Study the drawing (mm; zero at the part's minimum x, y, z) and answer. Give positions to 0.01 mm unless a question says otherwise; leave off trailing zeros. Loops run counter-clockwise (first coordinate to the right, second up) from the corner with the lowest first, then second, coordinate; pieces in that order, holes last. Notation, with made-up numbers: (-11.75, 30) - (22.25, 30) arc R12 cw to (22.25, 43) - close; hole circle Ø6 at (-39.5, -18.5). An arc over 180 degrees is marked (long way). Write item = value, one per line. Start each with the question number.
1) The part is cut by section B-B on x = 25.4. Write down the section's boundary in (y, z).
2) Flat-ended cylindrical pins translate along their axes: P1, Ø1, axis at x = 39, y = 3.5, coming from the -Z side; P2, Ø6, axis at x = 13.5, y = 12.5, coming from the +Z side; P3, Ø1.5, axis at y = 11.5, z = 26.5, coming from the -X side (1 decimal). Find the tip coordinate at first contact, or state that the pin passes through.
3) The mould has two halves that part along Y. Classify the marked faces 1, 2 and 3: +Y half, -Y half, draft (parallel to the pull), parting line (faces both ways), or undercut.
4) The part is cut by section A-A on z = 25.4. Write down the section's boundary in (x, y).
5) Consider probe 1 along Z at (x, y) = (28.5, 14.25); probe 2 along Z at (x, y) = (7.5, 8) (1 decimal); probe 3 along X at (y, z) = (8.75, 14.5) (1 decimal). Determine where each line is inside the solid, lowest interval first.
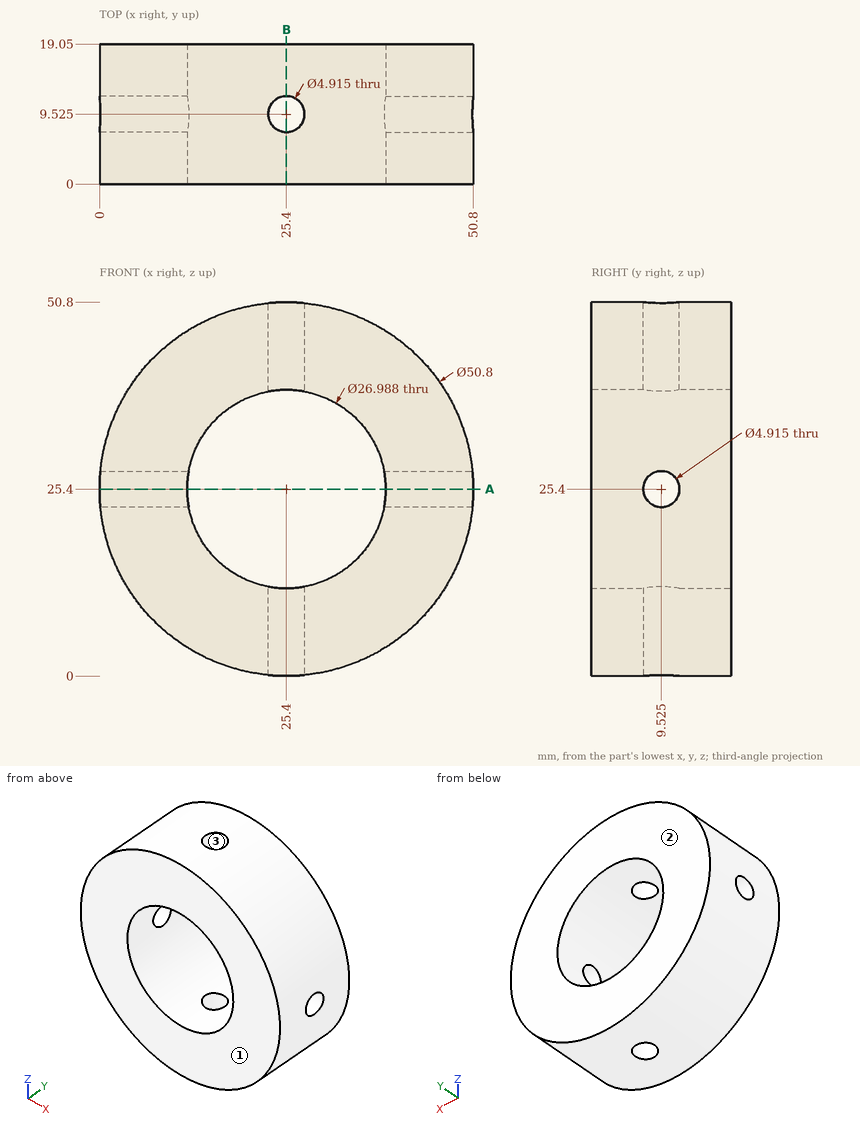
Answer below:
q1.outline = (0, 0) - (7.07, 0) - (7.07, 11.91) - (0, 11.91) - close; (0, 38.89) - (7.07, 38.89) - (7.07, 50.8) - (0, 50.8) - close; (11.98, 0) - (19.05, 0) - (19.05, 11.91) - (11.98, 11.91) - close; (11.98, 38.89) - (19.05, 38.89) - (19.05, 50.8) - (11.98, 50.8) - close
q2.P1 = 3.64
q2.P2 = 49.19
q2.P3 = 0
q3.face_1 = -Y half
q3.face_2 = +Y half
q3.face_3 = undercut
q4.outline = (0, 0) - (11.91, 0) - (11.91, 7.07) - (0, 7.07) - close; (0, 11.98) - (11.91, 11.98) - (11.91, 19.05) - (0, 19.05) - close; (38.89, 0) - (50.8, 0) - (50.8, 7.07) - (38.89, 7.07) - close; (38.89, 11.98) - (50.8, 11.98) - (50.8, 19.05) - (38.89, 19.05) - close
q5.probe_1 = 0.19 to 12.27, 38.53 to 50.61
q5.probe_2 = 7.4 to 23.5, 27.3 to 43.4
q5.probe_3 = 2.5 to 17.4, 33.4 to 48.3
